The model under review builds one solid part; all positions refer to its coordinate system, in mm. A direction names the side the tool comes from. Round coordinates to 2 decimals unless told otherwise and drop trailing zeros. Order: outer loops, then holes, each group sorted by start corner. A loop starts at its lowest first (then second) coordinate and runs counter-clockwise, first axis right, second up. Notation, with made-up numbers: M 53.5,53.5 L 71.5,53.5 A17 ccw 71.5,86.5 Z; hole C 35.25,10 d6. An arc over 180 degrees is marked long. Answer as a JSON object with one key per item and string values. Group by question number.
1. Add section D-D on x = -15.5. State the section outline as (y, z) points, and give its area (3 significant figures).
2. Add section C-C on y = 28. State the section outline as (x, z) points, and give its area (3 significant figures).
3. To check wall thickness, follow probe 1 along X at (y, z) = (5, 20.5); probe 2 along Y at (x, z) = (-13, -24); probe 3 along Z at (x, y) = (26, 26.5). State the ranges of each line that lie inside material, in increasing order. Write a range as [from, to].
4. Add section B-B on x = 1. State the section outline as (y, z) points, and give its area (3 significant figures).
5. Machinability: for faces 1 (the face through (30, 24, 0)), 2 (the face through (20.83, 68.26, -2.6)), which of the approach directions +Z, -Z, +X, -X, +Y, -Y give a long, thin tool a straight path to every point of the face, cutting with its end or side? Answer none if there is none.
6. Clearance check with flat-ended pins moving along their axes: P1, Ø2, axis at x = -12, z = -21, coming from the -Y side; P2, Ø1.6, axis at x = -31, y = 33, coming from the +Z side; P3, Ø0.8, axis at x = -30.5, y = 36.5, coming from the -Z side; P4, Ø1.2, axis at x = -31, z = -6, coming from the +Y side. State where each tip first meets the part, or that it passes through.
7. Add section A-A on z = 0. State the section outline as (x, y) points, and give its area (3 significant figures).
```python
from build123d import *

# Parameters (mm, degrees)
SKETCH_1_W      = 60
SKETCH_1_H      = 60
EXTRUDE_1_DEPTH = 51
SKETCH_2_R      = 20
EXTRUDE_2_DEPTH = 35
SKETCH_4_W      = 30
SKETCH_4_H      = 25
EXTRUDE_3_DEPTH = 2
FILLET_4_R      = 5
FILLET_5_R      = 0.5
FILLET_6_R      = 3


with BuildPart() as part:
    # 草圖1 → 填料-伸長1 (new body)
    with BuildSketch(Plane(origin=(0, 0, 0), x_dir=(1, 0, 0), z_dir=(0, 1, 0))):
        Rectangle(SKETCH_1_W, SKETCH_1_H)
    extrude(amount=EXTRUDE_1_DEPTH)

    # 草圖2 → 填料-伸長2 (add)
    with BuildSketch(Plane(origin=(0, 51, 0), x_dir=(1, 0, 0), z_dir=(0, 1, 0))):
        with Locations(Location((1, 0, 0), (0, 0, 270))):
            Circle(SKETCH_2_R)
    extrude(amount=EXTRUDE_2_DEPTH)

    # 草圖4 → 填料-伸長3 (add)
    with BuildSketch(Plane.ZY.offset(30)):
        with Locations((0, 32.5)):
            Rectangle(SKETCH_4_W, SKETCH_4_H)
    extrude(amount=EXTRUDE_3_DEPTH)

    # 圓角4
    fillet_4_edges = [part.edges().sort_by_distance(p)[0] for p in [
        (30, 25.5, 30),
        (-30, 25.5, 30),
        (-30, 25.5, -30),
        (30, 25.5, -30),
    ]]
    fillet(fillet_4_edges, radius=FILLET_4_R)

    # 圓角5
    fillet_5_edges = [part.edges().sort_by_distance(p)[0] for p in [
        (-32, 32.5, 15),
        (-32, 45, 0),
        (-32, 32.5, -15),
        (-32, 20, 0),
    ]]
    fillet(fillet_5_edges, radius=FILLET_5_R)

    # 圓角6
    fillet_6_edges = [part.edges().sort_by_distance(p)[0] for p in [
        (0, 51, -30),
        (30, 51, 0),
        (-30, 51, 0),
        (0, 51, 30),
        (-28.535533906, 51, 28.535533906),
        (-28.535533906, 51, -28.535533906),
        (28.535533906, 51, 28.535533906),
        (28.535533906, 51, -28.535533906),
    ]]
    fillet(fillet_6_edges, radius=FILLET_6_R)


solid = part.part
```
Recorded:
{
 "1": {"outline": "M 0,-30 L 48,-30 A3 ccw 51,-27 L 51,-11.3 L 86,-11.3 L 86,11.3 L 51,11.3 L 51,27 A3 ccw 48,30 L 0,30 Z", "area": "3,850 mm²"},
 "2": {"outline": "M -32,-14.5 A0.5 ccw -31.5,-15 L -30,-15 L -30,-25 A5 ccw -25,-30 L 25,-30 A5 ccw 30,-25 L 30,25 A5 ccw 25,30 L -25,30 A5 ccw -30,25 L -30,15 L -31.5,15 A0.5 ccw -32,14.5 Z", "area": "3,640 mm²"},
 "3": {"probe 1": "x = [-30, 30]", "probe 2": "y = [0, 51]", "probe 3": "z = [-29.9, 29.9]"},
 "4": {"outline": "M 0,-30 L 48,-30 A3 ccw 51,-27 L 51,-20 L 86,-20 L 86,20 L 51,20 L 51,27 A3 ccw 48,30 L 0,30 Z", "area": "4,460 mm²"},
 "5": {"face 1": "+Z, -Z, +X, +Y, -Y", "face 2": "+Y"},
 "6": {"P1": "stops at y = 0", "P2": "stops at z = 15", "P3": "stops at z = -15", "P4": "stops at y = 45"},
 "7": {"outline": "M -32,20.5 A0.5 ccw -31.5,20 L -30,20 L -30,0 L 30,0 L 30,48 A3 ccw 27,51 L 21,51 L 21,86 L -19,86 L -19,51 L -27,51 A3 ccw -30,48 L -30,45 L -31.5,45 A0.5 ccw -32,44.5 Z", "area": "4,510 mm²"}
}
